Verification items for the finished model (mm, model axes). Face numbers are marked on the shaded views. A direction names the side the tool comes from. Coordinates: 2 decimals unless noted, no trailing zeros. Loops run counter-clockwise (first coordinate to the right, second up) from the corner with the lowest first, then second, coordinate; pieces in that order, holes last. Notation, with made-up numbers: (66.5, -10.75) -> (89.5, -10.75) arc R9 ccw to (89.5, -2.75) -> close; hole circle Ø7 at (42, 20). An arc over 180 degrees is marked (long way). Answer as a JSON object with one key per item and string values. Group by question number.
Q1. Scan lines: L1, parallel to Y at x = -27.5, z = 38.5; L2, parallel to Z at x = -67, y = -25; L3, parallel to X at y = -21.5, z = 75. Record each from-to range of solid material in increasing order.
Q2. Release check for a two-part mould opening along X. For the marked faces 1, 2 and 3 record: released by +X, released by -X, zero draft, split by the parting line, or undercut.
Q3. Cross-section at B-B on y = -32. Record the boundary of the cut face in (x, z), and give its area (3 significant figures).
Q4. Set-up check for the marked faces 4, 5 and 6: record each of +Z, -Z, +X, -X, +Y, -Y from which the full face is reachable in a straight line by a thin tool's end or side.
Q5. Cross-section at A-A on x = -11.5. Record the boundary of the cut face in (y, z), and give its area (3 significant figures).
Q6. Gauge pin test, flat ends, axial feed: pin 1 Ø10 at (x, y) = (-34, -28.5) entering from -Z; pin 2 Ø2 at (y, z) = (-12, 84.5) entering from -X; pin 3 Ø8 at (x, y) = (11.5, -32.5) entering from +Z; pin 4 Ø1 at (x, y) = (-79.5, -17) entering from +Z. Record the tip position at first contact, or that the pin passes through.
Q7. Cross-section at D-D on x = 22. Record the boundary of the cut face in (y, z), and give its area (3 significant figures).
Q8. Cross-section at C-C on z = 47. Record the boundary of the cut face in (x, y), and give its area (3 significant figures).
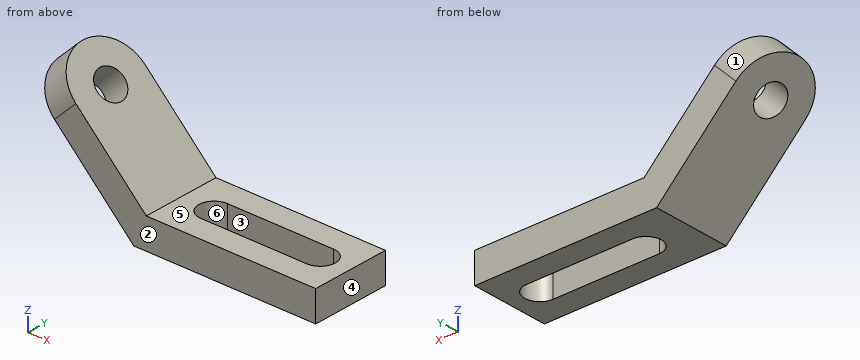
```python
from build123d import *

# Parameters (mm, degrees)
F1_DEPTH = 52
F2_R     = 25.99999
F4_DEPTH = 26
F5_R     = 10
F6_DEPTH = 25


# Not quite as in the source:
# - a fillet or chamfer is up to 0.001 mm smaller than in the source, because OpenCascade refuses the exact size


with BuildPart() as f1:
    # F0 (on Front) → F1 (new body)
    with BuildSketch(Plane.XZ):
        Polygon((-156.8951708629, 103.594939314), (-86.1844927443, 32.8842611954), (33.8155072557, 32.8842611954), (33.8155072557, 52.8842611954), (-77.9002214968, 52.8842611954), (-142.7530352392, 117.7370749377), align=None)
    extrude(amount=F1_DEPTH)

    # F2 (radius 26 in the source; OpenCascade refuses exactly that, so slightly less here)
    f2_edges = [f1.edges().sort_by_distance(p)[0] for p in [
        (-149.824103, -52, 110.666007),
        (-149.824103, 0, 110.666007),
    ]]
    fillet(f2_edges, radius=F2_R)

    # F3 (on face) → F4 (cut)
    with BuildSketch(Plane(origin=(0, 0, 32.8842611954), x_dir=(1, 0, 0), z_dir=(0, 0, -1))):
        with BuildLine():
            ThreePointArc((-56.184492662, 36), (-66.1844927443, 26), (-56.184492662, 16))
            Line((-56.184492662, 16), (13.8155072557, 16))
            ThreePointArc((13.8155072557, 16), (23.8155072557, 26), (13.8155072557, 36))
            Line((13.8155072557, 36), (-56.184492662, 36))
        make_face()
    extrude(amount=-F4_DEPTH, mode=Mode.SUBTRACT)

    # F5 (on face) → F6 (cut)
    with BuildSketch(Plane(origin=(-12.5079801507, 0, -12.5079801507), x_dir=(0.7071067812, 0, -0.7071067812), z_dir=(0.7071067812, 0, 0.7071067812))):
        with Locations((-158.1943233382, -26)):
            Circle(F5_R)
    extrude(amount=-F6_DEPTH, mode=Mode.SUBTRACT)


solid = f1.part
```
Computed values:
{
 "1": {"L1": "y = -52 to -36, -16 to 0", "L2": "z = 32.88 to 52.88", "L3": "x = -128.3 to -100.02"},
 "2": {"face 1": "released by -X", "face 2": "zero draft", "face 3": "undercut"},
 "3": {"outline": "(-156.4, 103.1) -> (-144.17, 90.87) -> (-130.03, 105.01) -> (-142.26, 117.24) -> close; (-132.85, 79.55) -> (-86.18, 32.88) -> (-64.18, 32.88) -> (-64.18, 52.88) -> (-77.9, 52.88) -> (-118.71, 93.7) -> close; (21.82, 32.88) -> (33.82, 32.88) -> (33.82, 52.88) -> (21.82, 52.88) -> close", "area": "2,180 mm²"},
 "4": {"face 4": "+Z, -Z, +X, +Y, -Y", "face 5": "+Z, +X, +Y, -Y", "face 6": "+Z, -Z"},
 "5": {"outline": "(-52, 32.88) -> (-36, 32.88) -> (-36, 52.88) -> (-52, 52.88) -> close; (-16, 32.88) -> (0, 32.88) -> (0, 52.88) -> (-16, 52.88) -> close", "area": "640 mm²"},
 "6": {"pin 1": "passes through", "pin 2": "stops at x = -138.8", "pin 3": "stops at z = 52.88", "pin 4": "stops at z = 54.98"},
 "7": {"outline": "(-52, 32.88) -> (-31.75, 32.88) -> (-31.75, 52.88) -> (-52, 52.88) -> close; (-20.25, 32.88) -> (0, 32.88) -> (0, 52.88) -> (-20.25, 52.88) -> close", "area": "810 mm²"},
 "8": {"outline": "(-100.3, -52) -> (33.82, -52) -> (33.82, 0) -> (-100.3, 0) -> close; hole (-56.18, -36) -> (13.82, -36) arc R10 ccw to (13.82, -16) -> (-56.18, -16) arc R10 ccw to start", "area": "5,260 mm²"}
}
